from build123d import *

# Parameters (mm, degrees)
F0_W     = 15
F0_H     = 15
F1_DEPTH = 8.6


with BuildPart() as f1:
    # F0 (on Top) → F1 (new body)
    with BuildSketch(Plane.XY):
        with Locations((-7.5, 13.519098)):
            Rectangle(F0_W, F0_H)
    extrude(amount=F1_DEPTH)

    # F2 (on face) → F3 (revolve)
    with BuildSketch(Plane.XY.offset(8.6)):
        with BuildLine():
            Line((-7.5, 8.752942), (-7.5, 18.752942))
            ThreePointArc((-7.5, 18.752942), (-12.5, 13.752942), (-7.5, 8.752942))
        make_face()
    revolve(axis=Axis((-7.5, 13.752942, 8.6), (0, -1, 0)))


solid = f1.part
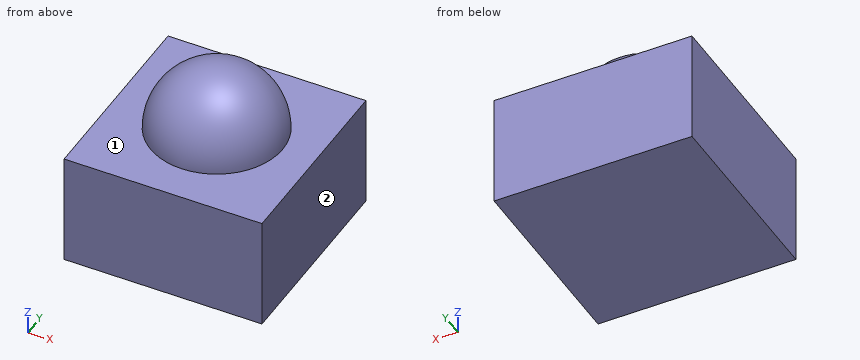
Model file for the job. Use its own axes, mm. Face numbers are marked on the shaded views. A direction names the side the tool comes from. Give positions to 0.01 mm unless a question says otherwise; leave off trailing zeros. Loops run counter-clockwise (first coordinate to the right, second up) from the corner with the lowest first, then second, coordinate; pieces in that order, holes last.
1) Saw through at D-D (x = -13.5). Write the cut outline in (y, z).
2) Wall check: line 1 (Z direction, x = -1.75, y = 15.5); line 2 (X direction, y = 11.25, z = 11.75); line 3 (Z direction, x = -8.5, y = 15.75). Give the ranges that are in metal, low to high.
3) Saw through at C-C (z = 12). Write the cut outline in (x, y), plus the area to 3 significant figures.
4) Tool access for the marked faces 1 and 2: list every direction of +Z, -Z, +X, -X, +Y, -Y with a clear straight run to the whole face (end or side of a thin tool).
5) Saw through at A-A (x = -3.25). Write the cut outline in (y, z).
6) Saw through at B-B (y = 10). Write the cut outline in (x, z).
Answer block:
1. outline: (6.02, 0) - (21.02, 0) - (21.02, 8.6) - (6.02, 8.6) - close
2. line 1: z = 0 to 8.6
2. line 2: x = -10.47 to -4.53
2. line 3: z = 0 to 13.07
3. outline: circle Ø7.33 at (-7.5, 13.75)
3. area: 42.2 mm2
4. face 1: +Z
4. face 2: +Z, -Z, +X, +Y, -Y
5. outline: (6.02, 0) - (21.02, 0) - (21.02, 8.6) - (16.39, 8.6) arc R2.63 ccw to (11.12, 8.6) - (6.02, 8.6) - close
6. outline: (-15, 0) - (0, 0) - (0, 8.6) - (-4.2, 8.6) arc R3.3 ccw to (-10.8, 8.6) - (-15, 8.6) - close
